from build123d import *

# Parameters (mm, degrees)
F1_DEPTH = 419
F3_DEPTH = 5
F4_R     = 5


with BuildPart() as f1:
    # F0 (on Front) → F1 (new body)
    with BuildSketch(Plane.XZ):
        Polygon((-55.5, 0), (0, 0), (55.5, 0), (55.5, 4.9), (52.4, 4.9), (52.4, 10.1), (55.5, 10.1), (55.5, 15), (52.4, 15), (52.4, 20), (0, 20), (-52.4, 20), (-52.4, 15), (-55.5, 15), (-55.5, 10.1), (-52.4, 10.1), (-52.4, 4.9), (-55.5, 4.9), align=None)
    extrude(amount=-F1_DEPTH)

    # F2 (on face) → F3 (cut)
    with BuildSketch(Plane.XY.offset(20)):
        Polygon((36.5, 385.258278), (-36.5, 385.258278), (-39, 310.258278), (39, 310.258278), align=None)
        Polygon((-36.5, 33.708609), (36.5, 33.708609), (39, 106.708609), (-39, 106.708609), align=None)
        Polygon((36.258278, 172.5), (36.258278, 245.5), (-38.741722, 248), (-38.741722, 170), align=None)
    extrude(amount=-F3_DEPTH, mode=Mode.SUBTRACT)

    # F4
    f4_edges = [f1.edges().sort_by_distance(p)[0] for p in [
        (-36.5, 385.258278, 17.5),
        (36.5, 385.258278, 17.5),
        (-39, 310.258278, 17.5),
        (39, 310.258278, 17.5),
        (-38.741722, 248, 17.5),
        (36.258278, 245.5, 17.5),
        (39, 106.708609, 17.5),
        (-39, 106.708609, 17.5),
        (-38.741722, 170, 17.5),
        (36.258278, 172.5, 17.5),
        (36.5, 33.708609, 17.5),
        (-36.5, 33.708609, 17.5),
    ]]
    fillet(f4_edges, radius=F4_R)


solid = f1.part
Read the model definition and answer for the solid it produces. Units are mm, in the model's axes. A direction names the side the tool comes from. Give positions to 0.01 mm unless a question says otherwise; leave off trailing zeros. Write each loop counter-clockwise with the first axis right and the second up, starting at its lowest first coordinate (ties: lowest second). Pieces come first, ordered by that corner, then holes. Notation, with made-up numbers: (-10, 62.5) - (0, 62.5) arc R22 ccw to (0, 101.5) - close; hole circle Ø1 at (64.25, 38). An arc over 180 degrees is marked (long way). Use CSV: the item, a comma, the result in double quotes. Start each with the question number.
(1) Find section A-A (y = 261). Give the vertices of the cut face in (x, z), plus the area to 3 significant figures.
(2) Find section C-C (y = 204). Give the vertices of the cut face in (x, z), plus the area to 3 significant figures.
(3) Find section B-B (x = 21.5). Give the vertices of the cut face in (y, z), plus the area to 3 significant figures.
(4) Find section D-D (y = 45). Give the vertices of the cut face in (x, z), plus the area to 3 significant figures.
(5) Determine the mould class of faces 1 (the flat face through (-1, 348, 15)), 2 (the flat face through (-1, 0, 10)) for opening direction X: +X half, -X half, draft (parallel to the pull), parting line (faces both ways), or undercut.
(6) For faces 3 (the flat face through (-1, 207, 0)), 4 (the flat face through (-1, 71, 15)), determine the directions among +Z, -Z, +X, -X, +Y, -Y from which every point of the face is accessible in a straight line to the end or side of a thin tool.
(7) Consider line 1 along Y through (x, z) = (22, 18.5); line 2 along X through (y, z) = (55.5, 8); line 3 along Z through (x, y) = (9, 235.5). Determine where each line is inside the solid, lowest interval first.
(8) Given P1, Ø1.5, axis at y = 282, z = 18, coming from the -X side; P2, Ø1.6, axis at x = 54.5, y = 247.5, coming from the +Z side; P3, Ø2.5, axis at y = 313, z = 18.5, coming from the +X side, each flat-ended and moving along its own axis, determine where each tip first touches the part or whether it passes through.
Findings below:
1,outline,"(-55.5, 0) - (55.5, 0) - (55.5, 4.9) - (52.4, 4.9) - (52.4, 10.1) - (55.5, 10.1) - (55.5, 15) - (52.4, 15) - (52.4, 20) - (-52.4, 20) - (-52.4, 15) - (-55.5, 15) - (-55.5, 10.1) - (-52.4, 10.1) - (-52.4, 4.9) - (-55.5, 4.9) - close"
1,area,"2,160 mm2"
2,outline,"(-55.5, 0) - (55.5, 0) - (55.5, 4.9) - (52.4, 4.9) - (52.4, 10.1) - (55.5, 10.1) - (55.5, 15) - (52.4, 15) - (52.4, 20) - (36.26, 20) - (36.26, 15) - (-38.74, 15) - (-38.74, 20) - (-52.4, 20) - (-52.4, 15) - (-55.5, 15) - (-55.5, 10.1) - (-52.4, 10.1) - (-52.4, 4.9) - (-55.5, 4.9) - close"
2,area,"1,780 mm2"
3,outline,"(0, 0) - (419, 0) - (419, 20) - (385.26, 20) - (385.26, 15) - (310.26, 15) - (310.26, 20) - (245.99, 20) - (245.99, 15) - (172.01, 15) - (172.01, 20) - (106.71, 20) - (106.71, 15) - (33.71, 15) - (33.71, 20) - (0, 20) - close"
3,area,"7,270 mm2"
4,outline,"(-55.5, 0) - (55.5, 0) - (55.5, 4.9) - (52.4, 4.9) - (52.4, 10.1) - (55.5, 10.1) - (55.5, 15) - (52.4, 15) - (52.4, 20) - (36.89, 20) - (36.89, 15) - (-36.89, 15) - (-36.89, 20) - (-52.4, 20) - (-52.4, 15) - (-55.5, 15) - (-55.5, 10.1) - (-52.4, 10.1) - (-52.4, 4.9) - (-55.5, 4.9) - close"
4,area,"1,790 mm2"
5,face 1,"undercut"
5,face 2,"draft"
6,face 3,"-Z, +X, -X, +Y, -Y"
6,face 4,"+Z"
7,line 1,"0 to 33.71, 106.71 to 172.02, 245.98 to 310.26, 385.26 to 419"
7,line 2,"-52.4 to 52.4"
7,line 3,"0 to 15"
8,P1,"x = -52.4"
8,P2,"z = 15"
8,P3,"x = 52.4"
